Geometry: see drawing. Coordinates: mm, zero at the bounding-box minimum. Give positions to 0.01 mm unless a question says otherwise; leave off trailing zeros. Write each loop counter-clockwise with the first axis right and the second up, starting at its lowest first coordinate (ties: lowest second). Pieces come first, ordered by that corner, then holes. Notation, with made-up numbers: (60.5, -15.75) -> (69.5, -15.75) arc R13 cw to (69.5, -8.75) -> close; hole circle Ø1 at (-33.75, -38). An arc over 180 degrees is marked (long way). Write item = value, one per line.
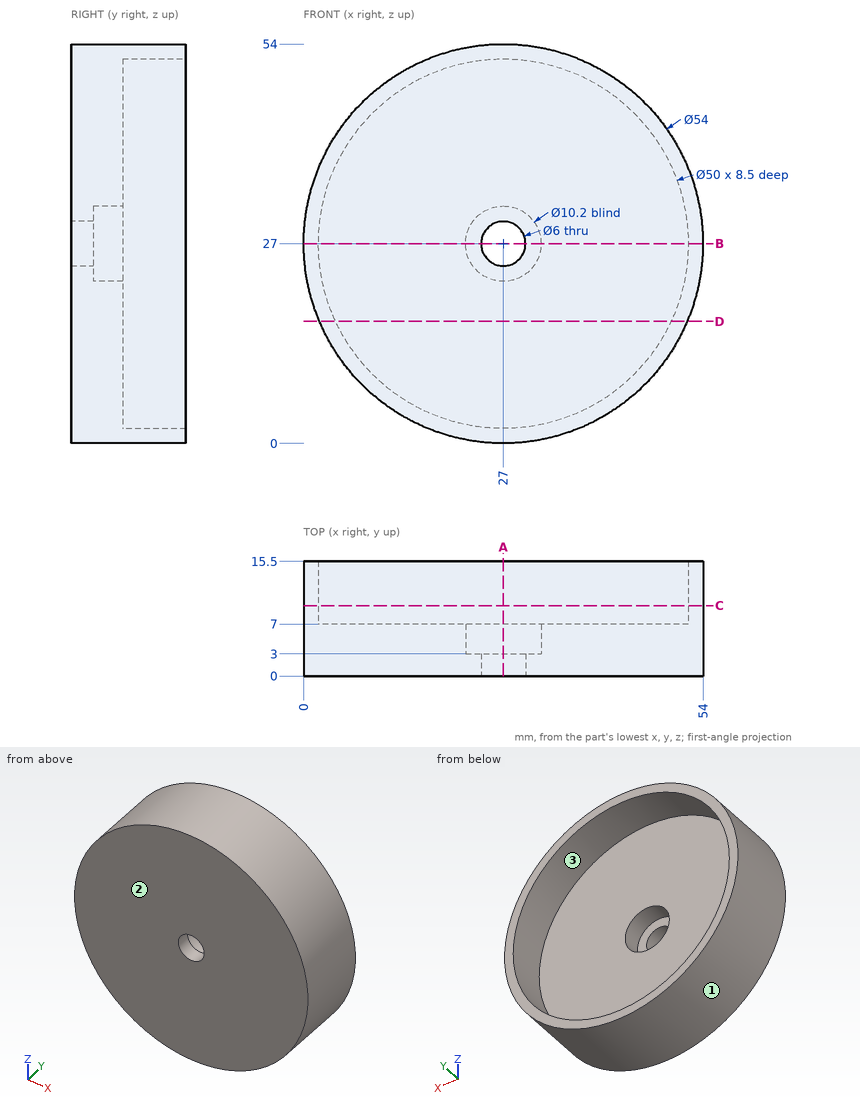
(1) Material intervals for line 1 (X direction, y = 1.7, z = 27); line 2 (X direction, y = 11, z = 27); line 3 (Y direction, x = 47, z = 35), sorted ascending.
Values follow:
line_1 = 0 to 24, 30 to 54
line_2 = 0 to 2, 52 to 54
line_3 = 0 to 7
(2) Section query D-D (z = 16.5). Return loops of the section in (x, y), plus the area to 3 significant figures.
Values follow:
outline = (2.13, 0) -> (51.87, 0) -> (51.87, 15.5) -> (49.69, 15.5) -> (49.69, 7) -> (4.31, 7) -> (4.31, 15.5) -> (2.13, 15.5) -> close
area = 385 mm2
(3) First-contact query: pin 1 (10 mm diameter, centred on x = 12, z = 22, fed in from +Y); pin 2 (1 mm diameter, centred on x = 35.5, y = 11, fed in from -Z); pin 3 (8 mm diameter, centred on y = 13.5, z = 45, fed in from +X). Flat tips, straight axial feed; report the tip coordinate or a pass-through.
Values follow:
pin_1 = 7
pin_2 = 1.21
pin_3 = 50.09
(4) Section query C-C (y = 9.5). Return loops of the section in (x, z).
Values follow:
outline = circle Ø54 at (27, 27); hole circle Ø50 at (27, 27)
(5) Pull-direction query (Z, two-part tool) for the marked faces 1, 2 and 3; classes: pulls with the +Z half, pulls with the -Z half, needs draft (parallel to the pull), parting line crosses it, or undercut.
Values follow:
face_1 = parting line crosses it
face_2 = needs draft
face_3 = undercut
(6) Section query B-B (z = 27). Return loops of the section in (x, y).
Values follow:
outline = (0, 0) -> (24, 0) -> (24, 3) -> (21.9, 3) -> (21.9, 7) -> (2, 7) -> (2, 15.5) -> (0, 15.5) -> close; (30, 0) -> (54, 0) -> (54, 15.5) -> (52, 15.5) -> (52, 7) -> (32.1, 7) -> (32.1, 3) -> (30, 3) -> close
(7) Section query A-A (x = 27). Return loops of the section in (y, z), plus the area to 3 significant figures.
Values follow:
outline = (0, 0) -> (15.5, 0) -> (15.5, 2) -> (7, 2) -> (7, 21.9) -> (3, 21.9) -> (3, 24) -> (0, 24) -> close; (0, 30) -> (3, 30) -> (3, 32.1) -> (7, 32.1) -> (7, 52) -> (15.5, 52) -> (15.5, 54) -> (0, 54) -> close
area = 353 mm2
